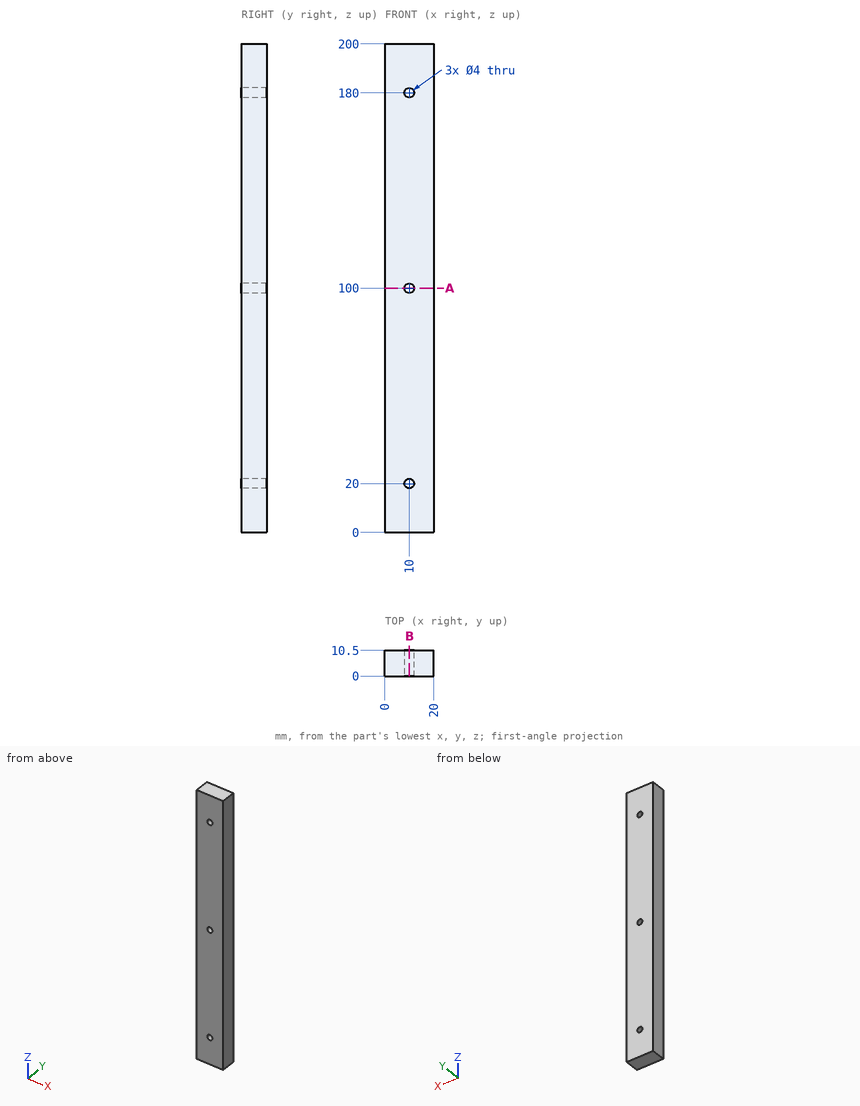
Geometry check sheet. Reference: drawing and pictorial views, mm from the part's lowest x, y, z. Round coordinates to 2 decimals unless told otherwise and drop trailing zeros. Write each loop counter-clockwise with the first axis right and the second up, starting at its lowest first coordinate (ties: lowest second). Pieces come first, ordered by that corner, then holes.
Item 1: Go/stop test with a flat-tipped pin: pin 1 Ø2.5 at (x, z) = (10, 100) entering from +Y. Record where the tip stops, or that it passes through.
Determined:
pin 1: passes through
Item 2: Section check A-A (z = 100). Record the boundary of the cut face in (x, y), plus the area to 3 significant figures.
Determined:
outline: (0, 0) - (8, 0) - (8, 10.5) - (0, 10.5) - close; (12, 0) - (20, 0) - (20, 10.5) - (12, 10.5) - close
area: 168 mm2
Item 3: Section check B-B (x = 10). Record the boundary of the cut face in (y, z), plus the area to 3 significant figures.
Determined:
outline: (0, 0) - (10.5, 0) - (10.5, 18) - (0, 18) - close; (0, 22) - (10.5, 22) - (10.5, 98) - (0, 98) - close; (0, 102) - (10.5, 102) - (10.5, 178) - (0, 178) - close; (0, 182) - (10.5, 182) - (10.5, 200) - (0, 200) - close
area: 1,970 mm2
Item 4: Material ranges on line 1 along Z through (x, y) = (9.75, 3.75); line 2 along X through (y, z) = (3.75, 180); line 3 along Z through (x, y) = (9, 1.75), recorded low to high.
Determined:
line 1: z = 0 to 18.02, 21.98 to 98.02, 101.98 to 178.02, 181.98 to 200
line 2: x = 0 to 8, 12 to 20
line 3: z = 0 to 18.27, 21.73 to 98.27, 101.73 to 178.27, 181.73 to 200
